The model under review builds one solid part; all positions refer to its coordinate system, in mm. Coordinates: 2 decimals unless noted, no trailing zeros. Order: outer loops, then holes, each group sorted by start corner. A loop starts at its lowest first (then second) coordinate and runs counter-clockwise, first axis right, second up. Notation, with made-up numbers: (0.5, 88.5) - (49.5, 88.5) arc R27 cw to (49.5, 104.5) - close; hole circle Ø1 at (-37, 51.25). An arc over 180 degrees is marked (long way). Answer in a Markdown table with one row per item.
```python
from build123d import *

# Parameters (mm, degrees)
SKETCH1_W           = 141.3
SKETCH1_H           = 60
SKETCH1_R           = 0.85
SKETCH1_R_2         = 5
BOSS_EXTRUDE1_DEPTH = 3


with BuildPart() as part:
    # Sketch1 → Boss-Extrude1 (new body)
    with BuildSketch(Plane.XY):
        Rectangle(SKETCH1_W, SKETCH1_H)
        with Locations((-68.15, 25)):
            Circle(SKETCH1_R, mode=Mode.SUBTRACT)
        with Locations(Location((-68.15, -25, 0), (0, 0, 180))):
            Circle(SKETCH1_R, mode=Mode.SUBTRACT)
        with Locations((68.15, -25)):
            Circle(SKETCH1_R, mode=Mode.SUBTRACT)
        with Locations(Location((68.15, 25, 0), (0, 0, 180))):
            Circle(SKETCH1_R, mode=Mode.SUBTRACT)
        with Locations((0, -10)):
            Circle(SKETCH1_R_2, mode=Mode.SUBTRACT)
        with Locations((-40, -10)):
            Circle(SKETCH1_R_2, mode=Mode.SUBTRACT)
        with Locations(Location((40, -10, 0), (0, 0, 180))):
            Circle(SKETCH1_R_2, mode=Mode.SUBTRACT)
        with Locations((40, 10)):
            Circle(SKETCH1_R_2, mode=Mode.SUBTRACT)
        with Locations(Location((0, 10, 0), (0, 0, 180))):
            Circle(SKETCH1_R_2, mode=Mode.SUBTRACT)
        with Locations(Location((-40, 10, 0), (0, 0, 180))):
            Circle(SKETCH1_R_2, mode=Mode.SUBTRACT)
    extrude(amount=BOSS_EXTRUDE1_DEPTH)


solid = part.part
```
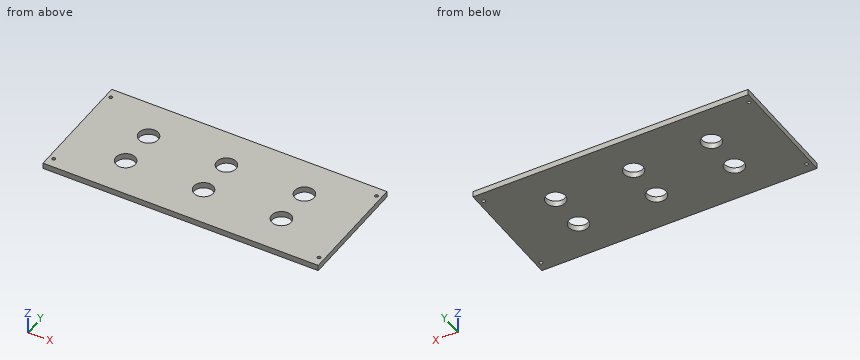
Item 1: Clearance check with a flat-ended pin moving along its axis: pin 1 Ø16 at (x, y) = (-40, 10) entering from -Z. State where the tip first meets the part, or that it passes through.
Check values:
| item | result |
|---|---|
| pin 1 | z = 0 |
Item 2: We need section A-A, the plane x = -40. Write out the cut boundary in (y, z).
Check values:
| item | result |
|---|---|
| outline | (-30, 0) - (-15, 0) - (-15, 3) - (-30, 3) - close; (-5, 0) - (5, 0) - (5, 3) - (-5, 3) - close; (15, 0) - (30, 0) - (30, 3) - (15, 3) - close |
Item 3: To check wall thickness, follow line 1 (Y direction, x = -40, z = 0.8); line 2 (Y direction, x = 68.15, z = 1.85); line 3 (X direction, y = -24.5, z = 1.8). State the ranges of each line that lie inside material, in increasing order. Write a range as from..to.
Check values:
| item | result |
|---|---|
| line 1 | -30..-15, -5..5, 15..30 |
| line 2 | -30..-25.85, -24.15..24.15, 25.85..30 |
| line 3 | -70.65..-68.84, -67.46..67.46, 68.84..70.65 |
Item 4: We need section B-B, the plane y = 10. Write out the cut boundary in (x, z), then the cut area to 3 significant figures.
Check values:
| item | result |
|---|---|
| outline | (-70.65, 0) - (-45, 0) - (-45, 3) - (-70.65, 3) - close; (-35, 0) - (-5, 0) - (-5, 3) - (-35, 3) - close; (5, 0) - (35, 0) - (35, 3) - (5, 3) - close; (45, 0) - (70.65, 0) - (70.65, 3) - (45, 3) - close |
| area | 334 mm^2 |
Item 5: We need section D-D, the plane x = -2.5. Write out the cut boundary in (y, z), then the cut area to 3 significant figures.
Check values:
| item | result |
|---|---|
| outline | (-30, 0) - (-14.33, 0) - (-14.33, 3) - (-30, 3) - close; (-5.67, 0) - (5.67, 0) - (5.67, 3) - (-5.67, 3) - close; (14.33, 0) - (30, 0) - (30, 3) - (14.33, 3) - close |
| area | 128 mm^2 |
Item 6: We need section C-C, the plane z = 1.1. State how many separate pieces and enclosed holes the cut face has, then the cut area to 3 significant figures.
Check values:
| item | result |
|---|---|
| separate pieces | 1 |
| enclosed holes | 10 |
| area | 8,000 mm^2 |
